CAD build for the part. Positions are in the model's coordinates, mm. A direction names the side the tool comes from. Give positions to 0.01 mm unless a question says otherwise; leave off trailing zeros. Write each loop counter-clockwise with the first axis right and the second up, starting at its lowest first coordinate (ties: lowest second). Pieces come first, ordered by that corner, then holes. Notation, with made-up numbers: (29.5, 42.5) -> (50.5, 42.5) arc R25 ccw to (50.5, 61.5) -> close; hole circle Ø6 at (24, -39.5). An arc over 180 degrees is marked (long way). Answer in a Markdown table with one row per item. Add a question column.
Autodesk Inventor part; units mm, degrees
ref_plane "YZ Plane" through (0, 0, 0) normal (1, 0, 0) x (0, 1, 0)
ref_plane "XZ Plane" through (0, 0, 0) normal (0, 1, 0) x (-1, 0, 0)
ref_plane "XY Plane" through (0, 0, 0) normal (0, 0, 1) x (1, 0, 0)
sketch "Sketch1" plane through (0, 0, 0) normal (0, 1, 0) x (-1, 0, 0)
  circle A0 centre (0, 0) radius 12.7
  circle A1 centre (0, 0) radius 31.75
  dimension "d0" = 25.4
  dimension "d1" = 63.5
extrude "Extrusion1" add sketch "Sketch1" along normal blind 12.7
sketch "Sketch2" plane through (0, 12.7, 0) normal (0, 1, 0) x (1, 0, 0)
  circle A0 centre (0, 0) radius 19.05
  circle A1 centre (0, 0) radius 31.75 construction
  line L0 (-31.75, 0) -> (-19.05, 0) construction
  circle A2 centre (-25.4, 0) radius 2.5473
  circle A3 centre (0, 0) radius 12.7
  dimension "d5" = 38.1
extrude "Extrusion2" add sketch "Sketch2" along normal blind 12.7 contours A0
sketch "Sketch3" plane through (0, 12.7, 0) normal (0, 1, 0) x (1, 0, 0)
  line L0 (-31.75, 0) -> (-19.05, 0) construction
  circle A0 centre (-25.4, 0) radius 2.5473
  point P0 (0, 0)
hole "Hole1" at (-25.4, 12.7, 0) direction (0, -1, 0) diameter 6.35 end through all
pattern_circular "Circular Pattern1" count 6 over 360 about axis through (0, 0, 0) along (0, 1, 0) of "Hole1"
sketch "Sketch4" plane through (0, 12.7, 0) normal (0, 1, 0) x (1, 0, 0)
  circle A0 centre (0, 0) radius 19.05
  line L0 (3.7235, -18.6826) -> (3.7235, -31.5309)
  arc A1 (-3.7247, -31.5309) -> (3.7235, -31.5309) centre (-0.0006, 0.0104) ccw
  line L1 (-3.7247, -31.5309) -> (-3.7247, -18.6823)
extrude "Extrusion3" add sketch "Sketch4" along normal blind 12.7 contours A0 L0 A1 L1
chamfer "Chamfer1" distance 12.7 angle 45 1 edges at (-0.0006, 25.4, 31.75)
pattern_circular "Circular Pattern2" count 6 over 360 about axis through (0, 0, 0) along (0, 1, 0) of "Extrusion3", "Chamfer1"
properties part number "pegg"
Item 1: Slice it at A-A, the plane y = 8.25. List the corners of the cut face in (x, z) (3 decimals), then the cut area to 3 significant figures.
Item 2: Mould opens along X. For faces 1 (the face through (6.883, 6.261, 30.995)), 2 (the face through (22.11, 18.96, 12.68)), 3 (the face through (0.837, 15.344, 12.672)), 4 (the face through (18.57, 17.55, -15.02)) say: released by +X, released by -X, zero draft, split by the parting line, or undercut.
Item 3: Drop flat-ended pins along their axis: pin 1 Ø5.5 at (x, z) = (12.7, -22) entering from +Y; pin 2 Ø3 at (y, z) = (17, -11) entering from +X; pin 3 Ø6 at (x, y) = (-5.5, 14) entering from -Z; pin 4 Ø5.5 at (x, z) = (-14.5, 19.5) entering from +Y. Give the stop position or say it passes through.
Item 4: Probe L1, parallel to X at y = 8.5, z = 0 (3 decimals); L2, parallel to X at y = 8, z = -22 (3 decimals); L3, parallel to Z at x = 15.5, y = 3. List the from-to ranges inside material, lowest first. Write a range as from..to.
Item 5: Slice it at B-B, the plane y = 17.25. List the corners of the cut face in (x, z), then the cut area to 3 significant figures.
Item 6: Which spindle directions (+Z, -Z, +X, -X, +Y, -Y) get a long thin tool onto all of the face, cutting with end or side? Do faces 5 (the face through (23, 12.7, -3)), 6 (the face through (-9.45, 18.96, 16.54)), 7 (the face through (9.45, 18.96, -16.54)). Say none if no direction does.
Answer key:
| question | item | result |
|---|---|---|
| 1 | outline | circle Ø63.5 at (0, 0); hole circle Ø6.35 at (-25.4, 0); hole circle Ø6.35 at (-12.7, -21.997); hole circle Ø6.35 at (-12.7, 21.997); hole circle Ø25.4 at (0, 0); hole circle Ø6.35 at (12.7, -21.997); hole circle Ø6.35 at (12.7, 21.997); hole circle Ø6.35 at (25.4, 0) |
| 1 | area | 2,470 mm² |
| 2 | face 1 | split by the parting line |
| 2 | face 2 | released by +X |
| 2 | face 3 | undercut |
| 2 | face 4 | undercut |
| 3 | pin 1 | passes through |
| 3 | pin 2 | stops at x = 26.72 |
| 3 | pin 3 | stops at z = -31.63 |
| 3 | pin 4 | stops at y = 12.7 |
| 4 | L1 | x = -31.75..-28.575, -22.225..-12.7, 12.7..22.225, 28.575..31.75 |
| 4 | L2 | x = -22.892..-15.875, -9.525..9.525, 15.875..22.892 |
| 4 | L3 | z = -27.71..-23.49, -20.5..20.5, 23.49..27.71 |
| 5 | outline | (-25.2, -10.25) arc R27.21 ccw to (-21.47, -16.7) -> (-14.32, -12.57) arc R19.05 ccw to (-3.72, -18.68) -> (-3.72, -26.94) arc R27.21 ccw to (3.72, -26.94) -> (3.72, -18.68) arc R19.05 ccw to (14.32, -12.57) -> (21.47, -16.7) arc R27.21 ccw to (25.2, -10.25) -> (18.04, -6.12) arc R19.05 ccw to (18.04, 6.12) -> (25.2, 10.25) arc R27.21 ccw to (21.47, 16.7) -> (14.32, 12.57) arc R19.05 ccw to (3.72, 18.68) -> (3.72, 26.94) arc R27.21 ccw to (-3.72, 26.94) -> (-3.72, 18.68) arc R19.05 ccw to (-14.32, 12.57) -> (-21.47, 16.7) arc R27.21 ccw to (-25.2, 10.25) -> (-18.04, 6.12) arc R19.05 ccw to (-18.04, -6.12) -> close; hole circle Ø25.4 at (0, 0) |
| 5 | area | 999 mm² |
| 6 | face 5 | +X, +Y |
| 6 | face 6 | +Z, +Y |
| 6 | face 7 | -Z, +Y |
